Source: three-view drawing plus pictorial views. Frame: mm from the lowest corner of the part. Coordinates: 2 decimals unless noted, no trailing zeros. Order: outer loops, then holes, each group sorted by start corner. A loop starts at its lowest first (then second) coordinate and runs counter-clockwise, first axis right, second up. Notation, with made-up numbers: (3, 57.5) -> (45, 57.5) arc R20 ccw to (45, 74.5) -> close; hole circle Ø8 at (13, -27). An arc over 180 degrees is marked (long way). Use one line per item in the form item = value. Start each with the question number.
1) Section query B-B on y = 1.4. Output: boundary loops of the cut face in (x, z).
2) Ray query, line 1 along Z through (x, y) = (8.5, 0.95); line 2 along Z through (x, y) = (9, 2) (1 decimal); line 3 along Z through (x, y) = (36.5, 1.65). Return the intervals inside material, ascending.
3) Section query A-A on x = 8.5. Output: boundary loops of the cut face in (y, z).
4) Pin query (flat end, axial travel): pin 1 (1.6 mm diameter, centred on y = 1.5, z = 99, fed in from -X); pin 2 (1.6 mm diameter, centred on x = 9, y = 2, fed in from -Z); pin 3 (1 mm diameter, centred on y = 1.5, z = 2, fed in from +X). Return the tip coordinate at first contact, or that it passes through.
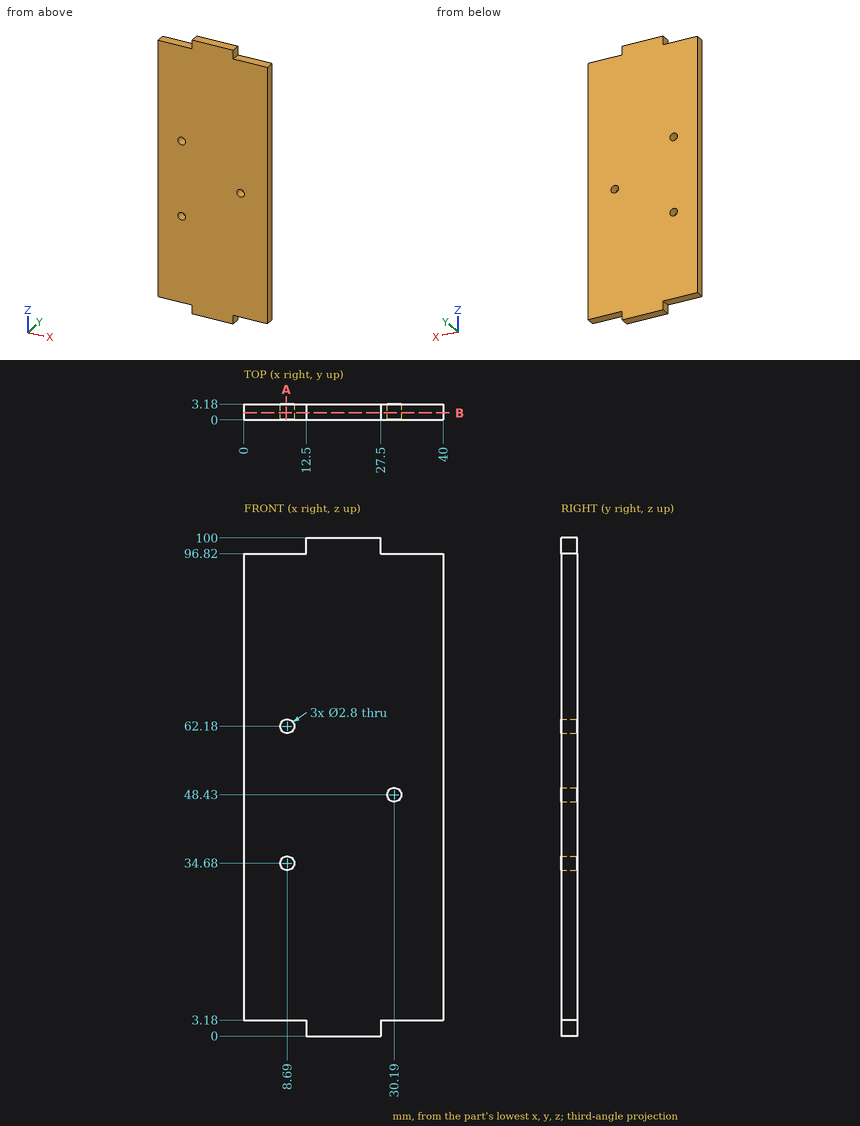
Answers below:
q1.outline = (0, 3.18) -> (12.5, 3.18) -> (12.5, 0) -> (27.5, 0) -> (27.5, 3.18) -> (40, 3.18) -> (40, 96.82) -> (27.5, 96.82) -> (27.5, 100) -> (12.5, 100) -> (12.5, 96.82) -> (0, 96.82) -> close; hole circle Ø2.8 at (8.69, 34.68); hole circle Ø2.8 at (8.69, 62.18); hole circle Ø2.8 at (30.19, 48.43)
q2.line_1 = 3.18 to 33.29, 36.07 to 60.79, 63.57 to 96.82
q2.line_2 = 3.2 to 33.3, 36 to 60.8, 63.5 to 96.8
q2.line_3 = 3.18 to 96.82
q3.outline = (0, 3.18) -> (3.18, 3.18) -> (3.18, 33.29) -> (0, 33.29) -> close; (0, 36.07) -> (3.18, 36.07) -> (3.18, 60.79) -> (0, 60.79) -> close; (0, 63.57) -> (3.18, 63.57) -> (3.18, 96.82) -> (0, 96.82) -> close
q4.pin_1 = 12.5
q4.pin_2 = 3.18
q4.pin_3 = 27.5
